```python
from build123d import *

# Parameters (mm, degrees)
SKETCH1_R           = 1.5
BOSS_EXTRUDE1_DEPTH = 4
SKETCH2_R           = 3.5
SKETCH2_R_2         = 1.5
CUT_EXTRUDE1_DEPTH  = 4
SKETCH3_W           = 4
SKETCH3_H           = 30
BOSS_EXTRUDE2_DEPTH = 3
SKETCH5_W           = 1.55
SKETCH5_H           = 2.6
SKETCH5_H_2         = 1.9
SKETCH5_H_3         = 5.5
SKETCH5_W_2         = 1.25
CUT_EXTRUDE2_DEPTH  = 10


with BuildPart() as part:
    # Sketch1 → Boss-Extrude1 (new body)
    with BuildSketch(Plane(origin=(0, 0, 0), x_dir=(0, 0, -1), z_dir=(1, 0, 0))):
        Polygon((30, 74), (20, 74), (20, 70), (10, 70), (10, 74), (0, 74), (0, 47), (4, 47), (4, 27), (0, 27), (0, 0), (10, 0), (10, 4), (20, 4), (20, 0), (30, 0), (30, 27), (26, 27), (26, 47), (30, 47), align=None)
        with Locations((2, 15)):
            Circle(SKETCH1_R, mode=Mode.SUBTRACT)
        with Locations((28, 15)):
            Circle(SKETCH1_R, mode=Mode.SUBTRACT)
        with Locations((2, 59)):
            Circle(SKETCH1_R, mode=Mode.SUBTRACT)
        with Locations((28, 59)):
            Circle(SKETCH1_R, mode=Mode.SUBTRACT)
    extrude(amount=BOSS_EXTRUDE1_DEPTH)

    # Sketch2 → Cut-Extrude1 (cut)
    with BuildSketch(Plane(origin=(4, 0, 0), x_dir=(0, 0, -1), z_dir=(1, 0, 0))):
        with Locations((15, 59)):
            Circle(SKETCH2_R)
        with Locations((7.928932188, 66.071067812)):
            Circle(SKETCH2_R_2)
        with Locations((22.071067812, 66.071067812)):
            Circle(SKETCH2_R_2)
        with Locations((22.071067812, 51.928932188)):
            Circle(SKETCH2_R_2)
        with Locations((7.928932188, 51.928932188)):
            Circle(SKETCH2_R_2)
    extrude(amount=-CUT_EXTRUDE1_DEPTH, mode=Mode.SUBTRACT)

    # Sketch3 → Boss-Extrude2 (add)
    with BuildSketch(Plane(origin=(0, 74, 0), x_dir=(1, 0, 0), z_dir=(0, 1, 0))):
        with Locations((2, 15)):
            Rectangle(SKETCH3_W, SKETCH3_H)
    extrude(amount=BOSS_EXTRUDE2_DEPTH)

    # Sketch5 → Cut-Extrude2 (cut)
    with BuildSketch(Plane(origin=(4, 0, 0), x_dir=(0, 0, -1), z_dir=(1, 0, 0))):
        with Locations((14.225, 12.7)):
            Rectangle(SKETCH5_W, SKETCH5_H)
        with Locations((14.225, 10.45)):
            Rectangle(SKETCH5_W, SKETCH5_H_2)
        with Locations((14.225, 6.75)):
            Rectangle(SKETCH5_W, SKETCH5_H_3)
        with Locations((15.775, 12.7)):
            Rectangle(SKETCH5_W, SKETCH5_H)
        with Locations((15.775, 10.45)):
            Rectangle(SKETCH5_W, SKETCH5_H_2)
        with Locations((15.775, 6.75)):
            Rectangle(SKETCH5_W, SKETCH5_H_3)
        with Locations((17.175, 10.45)):
            Rectangle(SKETCH5_W_2, SKETCH5_H_2)
        with Locations((12.825, 10.45)):
            Rectangle(SKETCH5_W_2, SKETCH5_H_2)
    extrude(amount=-CUT_EXTRUDE2_DEPTH, mode=Mode.SUBTRACT)


solid = part.part
```
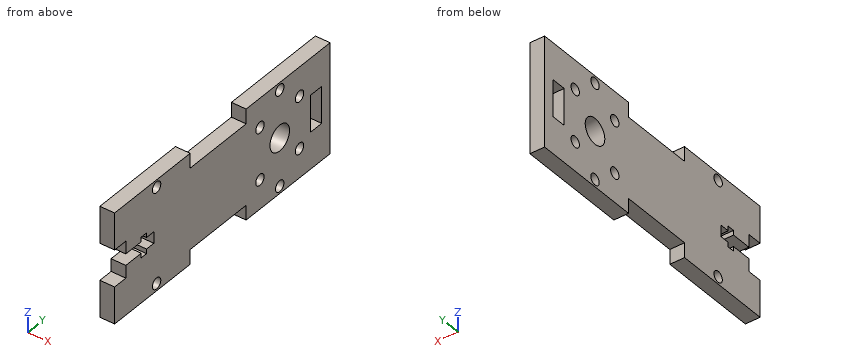
Design review of the part built by this model. Coordinates are the model's own, in mm. Coordinates: 2 decimals unless noted, no trailing zeros. Write each loop counter-clockwise with the first axis right and the second up, starting at its lowest first coordinate (ties: lowest second). Pieces come first, ordered by that corner, then holes.
1) Add section D-D (y = 59). Write out the cut boundary in (x, z).
2) Add section A-A (y = 15). Write out the cut boundary in (x, z), plus the area to 3 significant figures.
3) Insertion check: pin 1 (1 mm diameter, centred on x = 2, z = -12, fed in from -Y); pin 2 (1.8 mm diameter, centred on y = 66.07, z = -22.07, fed in from +X). Each pin has a flat end and moves straight along its axis. Give the tip position at first contact, or say it passes through.
4) Add section C-C (z = -2). Write out the cut boundary in (x, y).
5) To check wall thickness, follow L1, parallel to Y at x = 0.85, z = -2; L2, parallel to Y at x = 1.8, z = -14; L3, parallel to Y at x = 1.4, z = -18. State the ranges of each line that lie inside material, in increasing order.
6) Add section B-B (z = -15). Write out the cut boundary in (x, y).
Check result:
1. outline: (0, -30) - (4, -30) - (4, -29.5) - (0, -29.5) - close; (0, -26.5) - (4, -26.5) - (4, -18.5) - (0, -18.5) - close; (0, -11.5) - (4, -11.5) - (4, -3.5) - (0, -3.5) - close; (0, -0.5) - (4, -0.5) - (4, 0) - (0, 0) - close
2. outline: (0, -30) - (4, -30) - (4, -29.5) - (0, -29.5) - close; (0, -26.5) - (4, -26.5) - (4, -3.5) - (0, -3.5) - close; (0, -0.5) - (4, -0.5) - (4, 0) - (0, 0) - close
2. area: 96.0 mm2
3. pin 1: stops at y = 4
3. pin 2: passes through
4. outline: (0, 0) - (4, 0) - (4, 13.5) - (0, 13.5) - close; (0, 16.5) - (4, 16.5) - (4, 27) - (0, 27) - close; (0, 47) - (4, 47) - (4, 57.5) - (0, 57.5) - close; (0, 60.5) - (4, 60.5) - (4, 77) - (0, 77) - close
5. L1: y = 0 to 13.5, 16.5 to 27, 47 to 57.5, 60.5 to 77
5. L2: y = 14 to 55.65, 62.35 to 70, 74 to 77
5. L3: y = 4 to 57.2, 60.8 to 70, 74 to 77
6. outline: (0, 14) - (4, 14) - (4, 55.5) - (0, 55.5) - close; (0, 62.5) - (4, 62.5) - (4, 70) - (0, 70) - close; (0, 74) - (4, 74) - (4, 77) - (0, 77) - close
